from build123d import *

# Parameters (mm, degrees)
SKETCH1_W                      = 105
SKETCH1_H                      = 69
BOSS_EXTRUDE1_DEPTH            = 3.18
FILLET1_R                      = 3
SKETCH2_W                      = 105
SKETCH2_H                      = 91
BOSS_EXTRUDE2_DEPTH            = 15
FILLET2_R                      = 7
SKETCH3_W                      = 27
SKETCH3_H                      = 79
CUT_EXTRUDE1_DEPTH             = 0.25
SKETCH4_R                      = 0.79375
CUT_EXTRUDE2_DEPTH             = 0.25
MIRROR2_COPY_1_SKETCH_R        = 0.79375
MIRROR2_COPY_1_DEPTH           = 0.25
LPATTERN1_COUNT                = 3
LPATTERN1_PITCH                = 33
LPATTERN1_COPY_3_SKETCH_R      = 0.79375
LPATTERN1_COPY_3_DEPTH         = 0.25
LPATTERN1_COPY_4_SKETCH_R      = 0.79375
LPATTERN1_COPY_4_DEPTH         = 0.25
LPATTERN1_COPY_5_SKETCH_R      = 0.79375
LPATTERN1_COPY_5_DEPTH         = 0.25
LPATTERN1_COPY_6_SKETCH_R      = 0.79375
LPATTERN1_COPY_6_DEPTH         = 0.25
LPATTERN1_COPY_7_SKETCH_R      = 0.79375
LPATTERN1_COPY_7_DEPTH         = 0.25
LPATTERN1_COPY_8_SKETCH_R      = 0.79375
LPATTERN1_COPY_8_DEPTH         = 0.25
CBORE_FOR_M3_SHCS1_D           = 3.4
CBORE_FOR_M3_SHCS1_CBORE_D     = 6.5
CBORE_FOR_M3_SHCS1_CBORE_DEPTH = 4
MIRROR4_COPY_1_D               = 3.4
MIRROR4_COPY_1_CBORE_D         = 6.5
MIRROR4_COPY_1_CBORE_DEPTH     = 4
F_2_56_TAPPED_HOLE1_AT_2_COUNT = 2
F_2_56_TAPPED_HOLE1_AT_2_PITCH = 6
LPATTERN2_COUNT                = 3
LPATTERN2_PITCH                = 33


with BuildPart() as part:
    # Sketch1 → Boss-Extrude1 (new body)
    with BuildSketch(Plane(origin=(0, 0, 0), x_dir=(1, 0, 0), z_dir=(0, 1, 0))):
        Rectangle(SKETCH1_W, SKETCH1_H)
    extrude(amount=BOSS_EXTRUDE1_DEPTH)

    # Fillet1
    fillet1_edges = [part.edges().sort_by_distance(p)[0] for p in [
        (52.5, 1.59, 34.5),
        (-52.5, 1.59, 34.5),
        (-52.5, 1.59, -34.5),
        (52.5, 1.59, -34.5),
    ]]
    fillet(fillet1_edges, radius=FILLET1_R)

    # Sketch2 → Boss-Extrude2 (add)
    with BuildSketch(Plane(origin=(0, 3.18, 0), x_dir=(1, 0, 0), z_dir=(0, 1, 0))):
        Rectangle(SKETCH2_W, SKETCH2_H)
    extrude(amount=BOSS_EXTRUDE2_DEPTH)

    # Fillet2
    fillet2_edges = [part.edges().sort_by_distance(p)[0] for p in [
        (52.5, 10.68, 45.5),
        (52.5, 10.68, -45.5),
        (-52.5, 10.68, -45.5),
        (-52.5, 10.68, 45.5),
    ]]
    fillet(fillet2_edges, radius=FILLET2_R)

    # Sketch3 → Cut-Extrude1 (cut)
    with BuildSketch(Plane(origin=(0, 18.18, 0), x_dir=(1, 0, 0), z_dir=(0, 1, 0))):
        with Locations((-33, 0)):
            Rectangle(SKETCH3_W, SKETCH3_H)
    cut_extrude1 = extrude(amount=-CUT_EXTRUDE1_DEPTH, mode=Mode.SUBTRACT)

    # Sketch8 → #4-40 Tapped Hole1 (revolve, cut)
    with BuildSketch(Plane(origin=(-33, 18.18, -42.5), x_dir=(0, 0, 1), z_dir=(1, 0, 0))):
        Polygon((0, 0), (0, 7.679152758), (1.1303, 7), (1.1303, 0), align=None)
    f_4_40_tapped_hole1 = revolve(axis=Axis((-33, 24.53, -42.5), (0, -1, 0)), mode=Mode.SUBTRACT)

    # Mirror5: #4-40 Tapped Hole1 across plane
    add(f_4_40_tapped_hole1.mirror(Plane.XY), mode=Mode.SUBTRACT)

    # Sketch4 → Cut-Extrude2 (cut)
    with BuildSketch(Plane(origin=(0, 18.18, 0), x_dir=(1, 0, 0), z_dir=(0, 1, 0))):
        with Locations((-46.5, 39.5)):
            Circle(SKETCH4_R)
    cut_extrude2 = extrude(amount=-CUT_EXTRUDE2_DEPTH, mode=Mode.SUBTRACT)

    # Mirror1: Cut-Extrude2 across plane
    add(cut_extrude2.mirror(Plane(origin=(-33, 0, 0), x_dir=(0, 0, 1), z_dir=(1, 0, 0))), mode=Mode.SUBTRACT)

    # Mirror2: Cut-Extrude2 across plane
    add(cut_extrude2.mirror(Plane.XY), mode=Mode.SUBTRACT)

    # Mirror2 copy 1 sketch → Mirror2 copy 1 (cut)
    with BuildSketch(Plane(origin=(-66, 18.18, 0), x_dir=(-1, 0, 0), z_dir=(0, 1, 0))):
        with Locations((-46.5, 39.5)):
            Circle(MIRROR2_COPY_1_SKETCH_R)
    extrude(amount=-MIRROR2_COPY_1_DEPTH, mode=Mode.SUBTRACT)

    # LPattern1: Cut-Extrude1, #4-40 Tapped Hole1, Cut-Extrude2 ×3
    with Locations(*[(i * LPATTERN1_PITCH, 0, 0) for i in range(1, LPATTERN1_COUNT)]):
        add(cut_extrude1, mode=Mode.SUBTRACT)
        add(f_4_40_tapped_hole1, mode=Mode.SUBTRACT)
        add(cut_extrude2, mode=Mode.SUBTRACT)

    # LPattern1 copy 1 sketch → LPattern1 copy 1 (revolve, cut)
    with BuildSketch(Plane(origin=(0, 18.18, 42.5), x_dir=(0, 0, -1), z_dir=(1, 0, 0))):
        Polygon((0, 0), (0, -7.679152758), (1.1303, -7), (1.1303, 0), align=None)
    revolve(axis=Axis((0, 24.53, 42.5), (0, 1, 0)), mode=Mode.SUBTRACT)

    # LPattern1 copy 2 sketch → LPattern1 copy 2 (revolve, cut)
    with BuildSketch(Plane(origin=(33, 18.18, 42.5), x_dir=(0, 0, -1), z_dir=(1, 0, 0))):
        Polygon((0, 0), (0, -7.679152758), (1.1303, -7), (1.1303, 0), align=None)
    revolve(axis=Axis((33, 24.53, 42.5), (0, 1, 0)), mode=Mode.SUBTRACT)

    # LPattern1 copy 3 sketch → LPattern1 copy 3 (cut)
    with BuildSketch(Plane(origin=(-33, 18.18, 0), x_dir=(-1, 0, 0), z_dir=(0, 1, 0))):
        with Locations((-46.5, -39.5)):
            Circle(LPATTERN1_COPY_3_SKETCH_R)
    extrude(amount=-LPATTERN1_COPY_3_DEPTH, mode=Mode.SUBTRACT)

    # LPattern1 copy 4 sketch → LPattern1 copy 4 (cut)
    with BuildSketch(Plane(origin=(0, 18.18, 0), x_dir=(-1, 0, 0), z_dir=(0, 1, 0))):
        with Locations((-46.5, -39.5)):
            Circle(LPATTERN1_COPY_4_SKETCH_R)
    extrude(amount=-LPATTERN1_COPY_4_DEPTH, mode=Mode.SUBTRACT)

    # LPattern1 copy 5 sketch → LPattern1 copy 5 (cut)
    with BuildSketch(Plane(origin=(33, 18.18, 0), x_dir=(1, 0, 0), z_dir=(0, 1, 0))):
        with Locations((-46.5, -39.5)):
            Circle(LPATTERN1_COPY_5_SKETCH_R)
    extrude(amount=-LPATTERN1_COPY_5_DEPTH, mode=Mode.SUBTRACT)

    # LPattern1 copy 6 sketch → LPattern1 copy 6 (cut)
    with BuildSketch(Plane(origin=(66, 18.18, 0), x_dir=(1, 0, 0), z_dir=(0, 1, 0))):
        with Locations((-46.5, -39.5)):
            Circle(LPATTERN1_COPY_6_SKETCH_R)
    extrude(amount=-LPATTERN1_COPY_6_DEPTH, mode=Mode.SUBTRACT)

    # LPattern1 copy 7 sketch → LPattern1 copy 7 (cut)
    with BuildSketch(Plane(origin=(-33, 18.18, 0), x_dir=(-1, 0, 0), z_dir=(0, 1, 0))):
        with Locations((-46.5, 39.5)):
            Circle(LPATTERN1_COPY_7_SKETCH_R)
    extrude(amount=-LPATTERN1_COPY_7_DEPTH, mode=Mode.SUBTRACT)

    # LPattern1 copy 8 sketch → LPattern1 copy 8 (cut)
    with BuildSketch(Plane(origin=(0, 18.18, 0), x_dir=(-1, 0, 0), z_dir=(0, 1, 0))):
        with Locations((-46.5, 39.5)):
            Circle(LPATTERN1_COPY_8_SKETCH_R)
    extrude(amount=-LPATTERN1_COPY_8_DEPTH, mode=Mode.SUBTRACT)

    # CBORE for M3 SHCS1 (through all)
    with Locations(Plane(origin=(0, 18.18, 0), x_dir=(1, 0, 0), z_dir=(0, 1, 0))):
        with Locations((16.5, -22)):
            cbore_for_m3_shcs1 = CounterBoreHole(CBORE_FOR_M3_SHCS1_D / 2, CBORE_FOR_M3_SHCS1_CBORE_D / 2, CBORE_FOR_M3_SHCS1_CBORE_DEPTH)

    # Mirror3: CBORE for M3 SHCS1 across plane
    add(cbore_for_m3_shcs1.mirror(Plane(origin=(0, 0, 0), x_dir=(0, 0, 1), z_dir=(1, 0, 0))), mode=Mode.SUBTRACT)

    # Mirror4: CBORE for M3 SHCS1 across plane
    add(cbore_for_m3_shcs1.mirror(Plane.XY), mode=Mode.SUBTRACT)

    # Mirror4 copy 1 (through all)
    with Locations(Plane(origin=(0, 18.18, 0), x_dir=(-1, 0, 0), z_dir=(0, 1, 0))):
        with Locations((16.5, -22)):
            CounterBoreHole(MIRROR4_COPY_1_D / 2, MIRROR4_COPY_1_CBORE_D / 2, MIRROR4_COPY_1_CBORE_DEPTH)

    # Sketch10 → #2-56 Tapped Hole1 (revolve, cut)
    with BuildSketch(Plane(origin=(-30, 12.18, -45.5), x_dir=(0, 1, 0), z_dir=(1, 0, 0))):
        Polygon((0, 0), (0, 6.26416509), (0.889, 5.73), (0.889, 0), align=None)
    f_2_56_tapped_hole1 = revolve(axis=Axis((-30, 12.18, -51.85), (0, 0, 1)), mode=Mode.SUBTRACT)

    # #2-56 Tapped Hole1 at 2: #2-56 Tapped Hole1 ×2
    with Locations(*[(-i * F_2_56_TAPPED_HOLE1_AT_2_PITCH, 0, 0) for i in range(1, F_2_56_TAPPED_HOLE1_AT_2_COUNT)]):
        add(f_2_56_tapped_hole1, mode=Mode.SUBTRACT)

    # LPattern2: #2-56 Tapped Hole1 ×3
    with Locations(*[(i * LPATTERN2_PITCH, 0, 0) for i in range(1, LPATTERN2_COUNT)]):
        add(f_2_56_tapped_hole1, mode=Mode.SUBTRACT)

    # LPattern2 copy 1 sketch → LPattern2 copy 1 (revolve, cut)
    with BuildSketch(Plane(origin=(-3, 12.18, -45.5), x_dir=(0, 1, 0), z_dir=(1, 0, 0))):
        Polygon((0, 0), (0, 6.26416509), (0.889, 5.73), (0.889, 0), align=None)
    revolve(axis=Axis((-3, 12.18, -51.85), (0, 0, 1)), mode=Mode.SUBTRACT)

    # LPattern2 copy 2 sketch → LPattern2 copy 2 (revolve, cut)
    with BuildSketch(Plane(origin=(30, 12.18, -45.5), x_dir=(0, 1, 0), z_dir=(1, 0, 0))):
        Polygon((0, 0), (0, 6.26416509), (0.889, 5.73), (0.889, 0), align=None)
    revolve(axis=Axis((30, 12.18, -51.85), (0, 0, 1)), mode=Mode.SUBTRACT)


solid = part.part
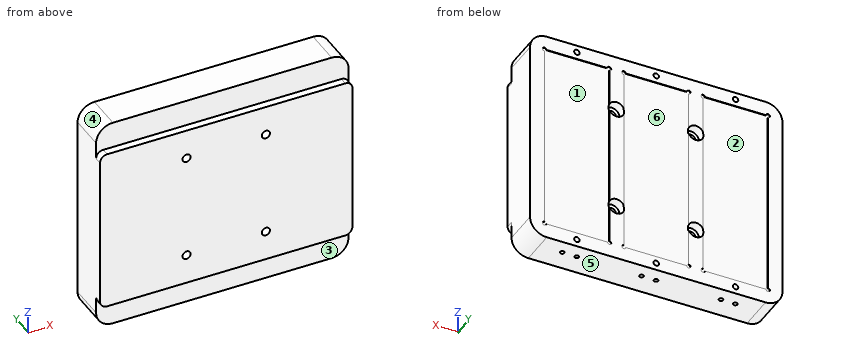
Work out the finished part from the listing and answer in its coordinate system (mm). Face numbers are marked on the shaded views. A direction names the side the tool comes from. Coordinates: 2 decimals unless noted, no trailing zeros. Loops run counter-clockwise (first coordinate to the right, second up) from the corner with the lowest first, then second, coordinate; pieces in that order, holes last. Notation, with made-up numbers: M 73.5,-10 L 79.5,-10 A29 cw 79.5,22 Z; hole C -25,-30.5 d7. An arc over 180 degrees is marked long. Answer in a Markdown table with one row per item. Add a question column.
1. Consider L1, parallel to Z at x = 16.5, y = 15.65; L2, parallel to Y at x = -3, z = -42.4; L3, parallel to Z at x = 18, y = 12. Determine where each line is inside the solid, lowest interval first.
2. The mould has two halves that part along Z. Classify the marked faces 1, 2, 3 and 4: pulls with the +Z half, pulls with the -Z half, needs draft (parallel to the pull), parting line crosses it, or undercut.
3. A tool of negligible diameter and unlimited length cuts with its end or side. For the marked faces 5 and 6, from which of +Z, -Z, +X, -X, +Y, -Y can it reach the whole face along a straight path? Write none if from no direction.
4. Find section A-A, the plane x = -16.5. Write down the section's boundary in (y, z), then the cut area to 3 significant figures.
5. Flat-ended cylindrical pins translate along their axes: P1, Ø5.5, axis at x = 16.5, z = -22, coming from the +Y side; P2, Ø7, axis at x = 8, z = 37.5, coming from the -Y side; P3, Ø1.8, axis at x = 0, z = 42.5, coming from the -Y side; P4, Ø4, axis at x = -26, z = -5, coming from the +Y side. Find the tip coordinate at first contact, or state that the pin passes through.
Reported:
| question | item | result |
|---|---|---|
| 1 | L1 | z = -45.5 to -25.25, -18.75 to 18.75, 25.25 to 45.5 |
| 1 | L2 | y = 3.18 to 11.29, 13.07 to 18.18 |
| 1 | L3 | z = -45.5 to -22.8, -21.2 to 21.2, 22.8 to 45.5 |
| 2 | face 1 | undercut |
| 2 | face 2 | undercut |
| 2 | face 3 | needs draft |
| 2 | face 4 | pulls with the +Z half |
| 3 | face 5 | -Z, +X, -X, +Y, -Y |
| 3 | face 6 | +Y |
| 4 | outline | M 0,-34.5 L 3.18,-34.5 L 3.18,-45.5 L 18.18,-45.5 L 18.18,-25.25 L 14.18,-25.25 L 14.18,-23.7 L 0,-23.7 Z; M 0,-20.3 L 14.18,-20.3 L 14.18,-18.75 L 18.18,-18.75 L 18.18,18.75 L 14.18,18.75 L 14.18,20.3 L 0,20.3 Z; M 0,23.7 L 14.18,23.7 L 14.18,25.25 L 18.18,25.25 L 18.18,45.5 L 3.18,45.5 L 3.18,34.5 L 0,34.5 Z |
| 4 | area | 1,440 mm^2 |
| 5 | P1 | stops at y = 14.18 |
| 5 | P2 | stops at y = 0 |
| 5 | P3 | stops at y = 3.18 |
| 5 | P4 | stops at y = 17.93 |
